Autodesk Fusion 360 part; units mm, degrees
sketch "草图1" plane through (0, 0, 0) normal (0, 0, 1) x (1, 0, 0)
  line L0 (-122.5473, -24.9077) -> (-143.5473, -24.9077)
  line L1 (-143.5473, -24.9077) -> (-143.5473, -19.9077)
  line L2 (-143.5473, -19.9077) -> (-122.5473, -19.9077)
  line L3 (-122.5473, -19.9077) -> (-122.5473, -24.9077)
  line L4 (-146.0473, -17.4077) -> (-120.0473, -17.4077)
  line L5 (-120.0473, -17.4077) -> (-120.0473, -27.4077)
  line L6 (-120.0473, -27.4077) -> (-146.0473, -27.4077)
  line L7 (-146.0473, -27.4077) -> (-146.0473, -17.4077)
  line L8 (-146.0473, -17.4077) -> (-120.0473, -27.4077) construction
  line L9 (-120.0473, -17.4077) -> (-146.0473, -27.4077) construction
  point P0 (-133.0473, -22.4077)
  dimension "d1" = 21
  dimension "d2" = 5
  dimension "d3" = 26
  dimension "d4" = 10
extrude "拉伸1" add sketch "草图1" along normal blind 65
sketch "草图2" plane through (0, 0, 65) normal (0, 0, 1) x (-1, 0, 0)
  line L0 (143.5473, 19.9077) -> (122.5473, 19.9077)
  line L1 (122.5473, 19.9077) -> (122.5473, 24.9077)
  line L2 (122.5473, 24.9077) -> (143.5473, 24.9077)
  line L3 (143.5473, 24.9077) -> (143.5473, 19.9077)
  line L4 (146.0473, 27.4077) -> (120.0473, 27.4077)
  line L5 (120.0473, 27.4077) -> (120.0473, 17.4077)
  line L6 (120.0473, 17.4077) -> (146.0473, 17.4077)
  line L7 (146.0473, 17.4077) -> (146.0473, 27.4077)
  line L8 (120.0473, 27.4077) -> (146.0473, 27.4077)
  line L9 (146.0473, 27.4077) -> (146.0473, 17.4077)
  line L10 (146.0473, 17.4077) -> (120.0473, 17.4077)
  line L11 (120.0473, 17.4077) -> (120.0473, 27.4077)
extrude "拉伸2" add sketch "草图2" along normal blind 2.5 contours L0 L1 L2 L3 | L4 L5 L6 L7 L8 L9 L10 L11
fillet "圆角1" radius 5 1 edges at (-122.5473, -22.4077, 65)
fillet "圆角2" radius 5 1 edges at (-143.5473, -22.4077, 65)
fillet "圆角3" radius 5 1 edges at (-120.0473, -22.4077, 67.5)
fillet "圆角4" radius 5 1 edges at (-146.0473, -22.4077, 67.5)
fillet "圆角5" radius 1 5 edges at (-120.0473, -17.4077, 31.25) (-121.5118, -17.4077, 66.0355) (-133.0473, -17.4077, 67.5) (-144.5829, -17.4077, 66.0355) (-146.0473, -17.4077, 31.25)
fillet "圆角6" radius 1 5 edges at (-146.0473, -27.4077, 31.25) (-144.5829, -27.4077, 66.0355) (-133.0473, -27.4077, 67.5) (-121.5118, -27.4077, 66.0355) (-120.0473, -27.4077, 31.25)
Design review of the part built by this model. Coordinates are the model's own, in mm. A direction names the side the tool comes from. Coordinates: 2 decimals unless noted, no trailing zeros. Order: outer loops, then holes, each group sorted by start corner. A loop starts at its lowest first (then second) coordinate and runs counter-clockwise, first axis right, second up. Notation, with made-up numbers: (40, 29) -> (52, 29) arc R29 ccw to (52, 62) -> close; hole circle Ø8 at (74, 29.25). An arc over 180 degrees is marked (long way). One line per item, written item: value. Start each with the question number.
Q1. Take a section at A-A, the plane z = 58. State the section outline as (x, y) points, then the cut area to 3 significant figures.
Q2. Take a section at C-C, the plane y = -23.25. State the section outline as (x, z) points, then the cut area to 3 significant figures.
Q3. For probe 1 along X at (y, z) = (-22, 13); probe 2 along Y at (x, z) = (-138, 49.5); probe 3 along Z at (x, y) = (-133, -23.75), list the stretches that pass through material, from the lowest coordinate up.
Q4. Mouldability with a two-part tool opening along Y and no side actions: class faces 3 (the flat face through (-133, -24.908, 32)), 4 (the flat face through (-133, -27.408, 33)), 5 (the flat face through (-146.047, -22, 31)), 6 (the flat face through (-133, -19.908, 32)) as pulls with the +Y half, pulls with the -Y half, needs draft (parallel to the pull), parting line crosses it, or undercut.
Q5. Take a section at B-B, the plane x = -134.5. State the section outline as (y, z) points.
Q6. Insertion check: pin 1 Ø2.5 at (x, y) = (-132.5, -22) entering from -Z; pin 2 Ø1 at (x, y) = (-140, -21) entering from -Z. Each pin has a flat end and moves straight along its axis. Give the tip position at first contact, or say it passes through.
Q7. Tool access review of faces 1 (the flat face through (-122.547, -22, 30)), 2 (the flat face through (-133, -26, 0)): name each direction out of +Z, -Z, +X, -X, +Y, -Y from which nothing blocks a thin tool from reaching the whole face with its end or side.
Values follow:
1. outline: (-146.05, -26.41) arc R1 ccw to (-145.05, -27.41) -> (-121.05, -27.41) arc R1 ccw to (-120.05, -26.41) -> (-120.05, -18.41) arc R1 ccw to (-121.05, -17.41) -> (-145.05, -17.41) arc R1 ccw to (-146.05, -18.41) -> close; hole (-143.55, -24.91) -> (-122.55, -24.91) -> (-122.55, -19.91) -> (-143.55, -19.91) -> close
1. area: 154 mm2
2. outline: (-146.05, 0) -> (-143.55, 0) -> (-143.55, 60) arc R5 cw to (-138.55, 65) -> (-127.55, 65) arc R5 cw to (-122.55, 60) -> (-122.55, 0) -> (-120.05, 0) -> (-120.05, 62.5) arc R5 ccw to (-125.05, 67.5) -> (-141.05, 67.5) arc R5 ccw to (-146.05, 62.5) -> close
2. area: 390 mm2
3. probe 1: x = -146.05 to -143.55, -122.55 to -120.05
3. probe 2: y = -27.41 to -24.91, -19.91 to -17.41
3. probe 3: z = 65 to 67.5
4. face 3: undercut
4. face 4: pulls with the -Y half
4. face 5: needs draft
4. face 6: undercut
5. outline: (-27.41, 0) -> (-24.91, 0) -> (-24.91, 65) -> (-19.91, 65) -> (-19.91, 0) -> (-17.41, 0) -> (-17.41, 66.5) arc R1 ccw to (-18.41, 67.5) -> (-26.41, 67.5) arc R1 ccw to (-27.41, 66.5) -> close
6. pin 1: stops at z = 65
6. pin 2: stops at z = 64.6
7. face 1: -Z
7. face 2: -Z, +X, -X, +Y, -Y
